Autodesk Inventor part; units mm, degrees
ref_plane "YZ Plane" through (0, 0, 0) normal (1, 0, 0) x (0, 1, 0)
ref_plane "XZ Plane" through (0, 0, 0) normal (0, 1, 0) x (-1, 0, 0)
ref_plane "XY Plane" through (0, 0, 0) normal (0, 0, 1) x (1, 0, 0)
sketch "Sketch1" plane through (0, 0, 0) normal (0, 0, 1) x (1, 0, 0)
  line L0 (4.16, 21.78) -> (23.76, 21.78)
  line L1 (23.76, 21.78) -> (23.76, -23.52)
  line L2 (23.76, -23.52) -> (4.16, -23.52)
  line L3 (4.16, -23.52) -> (4.16, 21.78)
  line L4 (4.16, 21.78) -> (23.76, 21.78)
  line L5 (13.96, 21.78) -> (13.96, 11.78)
  circle A0 centre (13.96, 11.78) radius 3
  point P0 (0, 0)
  dimension "d0" = 45.3
  dimension "d1" = 19.6
  dimension "d2" = 10
  dimension "d3" = 6
extrude "Extrusion1" add sketch "Sketch1" along normal blind 39.6 contours A0 | L0 L1 L2 L3
sketch "Sketch2" plane through (0, 0, 0) normal (0, 0, -1) x (-1, 0, 0)
  line L0 (-23.76, 21.78) -> (-4.16, 21.78)
  line L1 (-23.76, 21.78) -> (-4.16, 21.78)
  line L2 (-13.96, 21.78) -> (-13.96, 11.78)
  circle A0 centre (-13.96, 11.78) radius 3
  point P0 (0, 0)
  dimension "d6" = 10
  dimension "d7" = 6
extrude "Extrusion2" add sketch "Sketch2" along normal blind 10
sketch "Sketch3" plane through (13.96, 11.78, -10) normal (0, 0, -1) x (-1, 0, 0)
  circle A0 centre (0, 0) radius 3
  circle A1 centre (0, 0) radius 3
  point P0 (13.96, -11.78)
extrude "Extrusion3" add sketch "Sketch3" along normal blind 4
properties part number "motor_basic"
Model file for the job. Use its own axes, mm. A direction names the side the tool comes from. Give positions to 0.01 mm unless a question says otherwise; leave off trailing zeros. Loops run counter-clockwise (first coordinate to the right, second up) from the corner with the lowest first, then second, coordinate; pieces in that order, holes last.
Item 1: Slice it at C-C (z = -8.5). Write the cut outline in (x, y), plus the area to 3 significant figures.
Check values:
outline: circle Ø6 at (13.96, 11.78)
area: 28.3 mm2
Item 2: Slice it at A-A (x = 13.96). Write the cut outline in (y, z).
Check values:
outline: (-23.52, 0) - (8.78, 0) - (8.78, -14) - (14.78, -14) - (14.78, 0) - (21.78, 0) - (21.78, 39.6) - (-23.52, 39.6) - close
Item 3: Slice it at B-B (y = 11.78). Write the cut outline in (x, z), plus the area to 3 significant figures.
Check values:
outline: (4.16, 0) - (10.96, 0) - (10.96, -14) - (16.96, -14) - (16.96, 0) - (23.76, 0) - (23.76, 39.6) - (4.16, 39.6) - close
area: 860 mm2
Item 4: Drop a flat-ended pin along its axis: P1, Ø2, axis at x = 11, y = -15.5, coming from the -Z side. Give the stop position or say it passes through.
Check values:
P1: stops at z = 0
Item 5: Slice it at D-D (y = 5.5). Write the cut outline in (x, z), plus the area to 3 significant figures.
Check values:
outline: (4.16, 0) - (23.76, 0) - (23.76, 39.6) - (4.16, 39.6) - close
area: 776 mm2
Item 6: Which spindle directions (+Z, -Z, +X, -X, +Y, -Y) get a long thin tool onto all of the face, cutting with end or side? Do faces 1 (the face through (12.35, 9.25, -6.9)), 2 (the face through (23.76, -1, 20)). Say none if no direction does.
Check values:
face 1: -Z
face 2: +Z, -Z, +X, +Y, -Y
Item 7: Drill centre line: line 1 along Z through (x, y) = (12.75, 0). Where is it in solid material? Low to high.
Check values:
line 1: z = 0 to 39.6
